CAD build for the part. Positions are in the model's coordinates, mm. A direction names the side the tool comes from. Round coordinates to 2 decimals unless told otherwise and drop trailing zeros. Order: outer loops, then holes, each group sorted by start corner. A loop starts at its lowest first (then second) coordinate and runs counter-clockwise, first axis right, second up. Notation, with made-up numbers: M 50,49 L 79,49 A21 ccw 79,68 Z; hole C 51.5,75.5 d8. An arc over 180 degrees is marked long. Answer as a JSON object with one key per item and string values.
```python
from build123d import *

# Parameters (mm, degrees)
SKETCH_1_W          = 21.5
SKETCH_1_H          = 34.5
EXTRUDE_2_DEPTH     = 11
FILLET_1_R          = 2
SKETCH_2_W          = 39.173485157
SKETCH_2_H          = 57.857292793
CUT_EXTRUDE_1_DEPTH = 1
SKETCH_3_W          = 21.5
SKETCH_3_H          = 10
EXTRUDE_3_DEPTH     = 3
SKETCH_4_W          = 36.577122412
SKETCH_4_H          = 60.487116615
CUT_EXTRUDE_2_DEPTH = 1
SKETCH_5_W          = 14.5
SKETCH_5_H          = 3
CUT_EXTRUDE_3_DEPTH = 11
SKETCH_6_W          = 14.5
SKETCH_6_H          = 3
CUT_EXTRUDE_4_DEPTH = 11
SKETCH_7_W          = 57.52189795
SKETCH_7_H          = 59.987072635
CUT_EXTRUDE_5_DEPTH = 1
SKETCH_8_W          = 21.5
SKETCH_8_H          = 34.5
EXTRUDE_4_DEPTH     = 1
FILLET_2_R          = 2
SKETCH_9_W          = 42.225742073
SKETCH_9_H          = 59.055369136
CUT_EXTRUDE_6_DEPTH = 1
SKETCH_10_W         = 4
SKETCH_10_H         = 2
SKETCH_10_H_2       = 3.79495429
CUT_EXTRUDE_8_DEPTH = 30
CUT_EXTRUDE_9_DEPTH = 30


with BuildPart() as part:
    # 草图1 → 凸台-拉伸2 (new body)
    with BuildSketch(Plane(origin=(0, 0, 0), x_dir=(1, 0, 0), z_dir=(0, 1, 0))):
        with BuildLine():
            Line((-13.732977682, 21.876274057), (7.767022318, 21.876274057))
            ThreePointArc((7.767022318, 21.876274057), (9.18123588, 21.290487619), (9.767022318, 19.876274057))
            Line((9.767022318, 19.876274057), (9.767022318, -28.623725943))
            ThreePointArc((9.767022318, -28.623725943), (9.18123588, -30.037939506), (7.767022318, -30.623725943))
            Line((7.767022318, -30.623725943), (-13.732977682, -30.623725943))
            ThreePointArc((-13.732977682, -30.623725943), (-15.147191244, -30.037939506), (-15.732977682, -28.623725943))
            Line((-15.732977682, -28.623725943), (-15.732977682, 19.876274057))
            ThreePointArc((-15.732977682, 19.876274057), (-15.147191244, 21.290487619), (-13.732977682, 21.876274057))
        make_face()
        with Locations((-2.982977682, -4.373725943)):
            Rectangle(SKETCH_1_W, SKETCH_1_H, mode=Mode.SUBTRACT)
    extrude(amount=EXTRUDE_2_DEPTH)

    # 圆角1
    fillet_1_edges = [part.edges().sort_by_distance(p)[0] for p in [
        (-15.147191244, 11, -21.290487619),
        (-15.732977682, 11, 4.373725943),
        (-15.147191244, 11, 30.037939506),
        (-2.982977682, 11, 30.623725943),
        (9.18123588, 11, 30.037939506),
        (9.767022318, 11, 4.373725943),
        (9.18123588, 11, -21.290487619),
        (-2.982977682, 11, -21.876274057),
    ]]
    fillet(fillet_1_edges, radius=FILLET_1_R - 0.0001)  # a hair under: the kernel refuses the full size

    # 草图2 → 切除-拉伸1 (cut)
    with BuildSketch(Plane(origin=(0, 11, 0), x_dir=(1, 0, 0), z_dir=(0, 1, 0))):
        with Locations((-2.456788303, -4.185742432)):
            Rectangle(SKETCH_2_W, SKETCH_2_H)
    extrude(amount=-CUT_EXTRUDE_1_DEPTH, mode=Mode.SUBTRACT)

    # 草图3 → 凸台-拉伸3 (add)
    with BuildSketch(Plane(origin=(0, 0, 0), x_dir=(-1, 0, 0), z_dir=(0, -1, 0))):
        with Locations((2.982977682, -16.623725943)):
            Rectangle(SKETCH_3_W, SKETCH_3_H)
        with Locations((2.982977682, 7.876274057)):
            Rectangle(SKETCH_3_W, SKETCH_3_H)
    extrude(amount=-EXTRUDE_3_DEPTH)

    # 草图4 → 切除-拉伸2 (cut)
    with BuildSketch(Plane(origin=(0, 10, 0), x_dir=(1, 0, 0), z_dir=(0, 1, 0))):
        with Locations((-2.114714468, -5.96144712)):
            Rectangle(SKETCH_4_W, SKETCH_4_H)
    extrude(amount=-CUT_EXTRUDE_2_DEPTH, mode=Mode.SUBTRACT)

    # 草图5 → 切除-拉伸3 (cut)
    with BuildSketch(Plane(origin=(-13.732977682, 0, 0), x_dir=(0, 0, -1), z_dir=(1, 0, 0))):
        with Locations((-4.373725943, 1.5)):
            Rectangle(SKETCH_5_W, SKETCH_5_H)
    extrude(amount=-CUT_EXTRUDE_3_DEPTH, mode=Mode.SUBTRACT)

    # 草图6 → 切除-拉伸4 (cut)
    with BuildSketch(Plane.ZY.offset(-7.767022318)):
        with Locations((4.373725943, 1.5)):
            Rectangle(SKETCH_6_W, SKETCH_6_H)
    extrude(amount=-CUT_EXTRUDE_4_DEPTH, mode=Mode.SUBTRACT)

    # 草图7 → 切除-拉伸5 (cut)
    with BuildSketch(Plane(origin=(0, 0, 0), x_dir=(-1, 0, 0), z_dir=(0, -1, 0))):
        with Locations((4.496549364, -6.319684839)):
            Rectangle(SKETCH_7_W, SKETCH_7_H)
    extrude(amount=-CUT_EXTRUDE_5_DEPTH, mode=Mode.SUBTRACT)

    # 草图8 → 凸台-拉伸4 (add)
    with BuildSketch(Plane(origin=(0, 9, 0), x_dir=(1, 0, 0), z_dir=(0, 1, 0))):
        with BuildLine():
            Line((9.767022318, -28.623725943), (9.767022318, 19.876274057))
            ThreePointArc((9.767022318, 19.876274057), (9.18123588, 21.290487619), (7.767022318, 21.876274057))
            Line((7.767022318, 21.876274057), (-13.732977682, 21.876274057))
            ThreePointArc((-13.732977682, 21.876274057), (-15.147191244, 21.290487619), (-15.732977682, 19.876274057))
            Line((-15.732977682, 19.876274057), (-15.732977682, -28.623725943))
            ThreePointArc((-15.732977682, -28.623725943), (-15.147191244, -30.037939506), (-13.732977682, -30.623725943))
            Line((-13.732977682, -30.623725943), (7.767022318, -30.623725943))
            ThreePointArc((7.767022318, -30.623725943), (9.18123588, -30.037939506), (9.767022318, -28.623725943))
        make_face()
        with Locations((-2.982977682, -4.373725943)):
            Rectangle(SKETCH_8_W, SKETCH_8_H, mode=Mode.SUBTRACT)
    extrude(amount=EXTRUDE_4_DEPTH)

    # 圆角2
    fillet_2_edges = [part.edges().sort_by_distance(p)[0] for p in [
        (9.767022318, 10, 4.373725943),
        (9.18123588, 10, -21.290487619),
        (-2.982977682, 10, -21.876274057),
        (-15.147191244, 10, -21.290487619),
        (-15.732977682, 10, 4.373725943),
        (-15.147191244, 10, 30.037939506),
        (-2.982977682, 10, 30.623725943),
        (9.18123588, 10, 30.037939506),
    ]]
    fillet(fillet_2_edges, radius=FILLET_2_R - 0.0001)  # a hair under: the kernel refuses the full size

    # 草图9 → 切除-拉伸6 (cut)
    with BuildSketch(Plane(origin=(0, 10, 0), x_dir=(1, 0, 0), z_dir=(0, 1, 0))):
        with Locations((1.20063142, -3.725323224)):
            Rectangle(SKETCH_9_W, SKETCH_9_H)
    extrude(amount=-CUT_EXTRUDE_6_DEPTH, mode=Mode.SUBTRACT)

    # 草图10 → 切除-拉伸8 (cut)
    with BuildSketch(Plane.ZY.offset(15.732977682)):
        with Locations((-16.876274057, 7)):
            Rectangle(SKETCH_10_W, SKETCH_10_H)
        with Locations((-16.876274057, 9.897477145)):
            Rectangle(SKETCH_10_W, SKETCH_10_H_2)
    extrude(amount=-CUT_EXTRUDE_8_DEPTH, mode=Mode.SUBTRACT)

    # 草图11 → 切除-拉伸9 (cut)
    with BuildSketch(Plane.ZY.offset(15.732977682)):
        Polygon((23.623725943, 8), (23.623725943, 14.233861669), (27.623725943, 14.233861669), (27.623725943, 8), (27.623725943, 6), (23.623725943, 6), align=None)
    extrude(amount=-CUT_EXTRUDE_9_DEPTH, mode=Mode.SUBTRACT)


solid = part.part
```
Item 1: Saw through at C-C on x = -7. List the corners of the cut face in (y, z), and give its area (3 significant figures).
Worked answers:
{"outline": "M 1,-21.88 L 8,-21.88 A2 ccw 9,-21.61 L 9,-18.88 L 6,-18.88 L 6,-14.88 L 9,-14.88 L 9,-12.88 L 3,-12.88 L 3,-2.88 L 1,-2.88 Z; M 1,11.62 L 3,11.62 L 3,21.62 L 9,21.62 L 9,23.62 L 6,23.62 L 6,27.62 L 9,27.62 L 9,30.36 A2 ccw 8,30.62 L 1,30.62 Z", "area": "160 mm2"}
Item 2: Saw through at B-B on z = 8.5. List the corners of the cut face in (x, y), and give its area (3 significant figures).
Worked answers:
{"outline": "M -15.73,3 L -13.73,3 L -13.73,9 L -15.47,9 A2 ccw -15.73,8 Z; M 7.77,3 L 9.77,3 L 9.77,8 A2 ccw 9.5,9 L 7.77,9 Z", "area": "23.8 mm2"}
Item 3: Saw through at D-D on z = -11. List the corners of the cut face in (x, y), and give its area (3 significant figures).
Worked answers:
{"outline": "M -15.73,1 L 9.77,1 L 9.77,8 A2 ccw 9.5,9 L 7.77,9 L 7.77,3 L -13.73,3 L -13.73,9 L -15.47,9 A2 ccw -15.73,8 Z", "area": "74.8 mm2"}
Item 4: Two-plate mould, pull along Z, no slides. Class faces 4 (the flat face through (-3, 7, 27.624)), 5 (the cylindrical face through (-3.13, 8.51, -21.81)), 6 (the flat face through (-15.733, 4, 4)): released by +Z, released by -Z, zero draft, split by the parting line, or undercut.
Worked answers:
{"face 4": "undercut", "face 5": "released by -Z", "face 6": "zero draft"}
Item 5: 3-axis set-ups, long thin cutter, end or side, ignore diameter. For faces 1 (the flat face through (-3, 8, -18.876)), 2 (the flat face through (9, 3, 4)), 3 (the flat face through (7.767, 6, 5)): which of +Z, -Z, +X, -X, +Y, -Y reach the whole face in a straight line?
Worked answers:
{"face 1": "+X, -X, +Y", "face 2": "+X, -X, -Y", "face 3": "+Y"}
Item 6: Saw through at A-A on y = 2. List the corners of the cut face in (x, z), and give its area (3 significant figures).
Worked answers:
{"outline": "M -15.73,-19.88 A2 ccw -13.73,-21.88 L 7.77,-21.88 A2 ccw 9.77,-19.88 L 9.77,-2.88 L -15.73,-2.88 Z; M -15.73,11.62 L 9.77,11.62 L 9.77,28.62 A2 ccw 7.77,30.62 L -13.73,30.62 A2 ccw -15.73,28.62 Z", "area": "966 mm2"}
Item 7: Wall check: line 1 along Z through (x, y) = (-11, 7.5); line 2 along X through (y, z) = (4.25, -5); line 3 along Z through (x, y) = (3.25, 2.5). Give the ranges that are in metal, low to high. Write a range as [from, to].
Worked answers:
{"line 1": "z = [-21.88, -18.88], [-14.88, -12.88], [21.62, 23.62], [27.62, 30.62]", "line 2": "x = [-15.73, -13.73], [7.77, 9.77]", "line 3": "z = [-21.88, -2.88], [11.62, 30.62]"}
Item 8: Drop flat-ended pins along their axis: pin 1 Ø5 at (x, z) = (-1.5, -7) entering from +Y; pin 2 Ø1.6 at (x, z) = (-15, 3) entering from -Y; pin 3 Ø1.2 at (x, z) = (3, -18) entering from +Y. Give the stop position or say it passes through.
Worked answers:
{"pin 1": "stops at y = 3", "pin 2": "stops at y = 3", "pin 3": "stops at y = 6"}
